Geometry: final body of the model. Coordinates: model frame, mm. Face numbers are marked on the shaded views. Give positions to 0.01 mm unless a question says otherwise; leave off trailing zeros. Loops run counter-clockwise (first coordinate to the right, second up) from the corner with the lowest first, then second, coordinate; pieces in that order, holes last.
1. Material intervals for line 1 along Y through (x, z) = (231, 31.5); line 2 along Z through (x, y) = (208, 17); line 3 along Y through (x, z) = (153.5, 22), sorted ascending.
2. Section C-C, the plane x = 138. Output: boundary loops of the cut face in (y, z), then the cut area to 3 significant figures.
3. First-contact query: P1, Ø8, axis at x = 198.77, y = 19.99, coming from the +Z side; P2, Ø7, axis at x = 132.5, z = 25, coming from the +Y side; P3, Ø22, axis at x = 86, y = 18.5, coming from the +Z side. Flat tips, straight axial feed; report the tip coordinate or a pass-through.
4. Draft query along Y for the marked faces 1, 2, 3 and 4. Return one class per face: +Y half, -Y half, draft (parallel to the pull), parting line (faces both ways), or undercut.
5. Section A-A, the plane x = 31.5. Output: boundary loops of the cut face in (y, z), then the cut area to 3 significant figures.
6. Section B-B, the plane z = 42. Output: boundary loops of the cut face in (x, y), then the cut area to 3 significant figures.
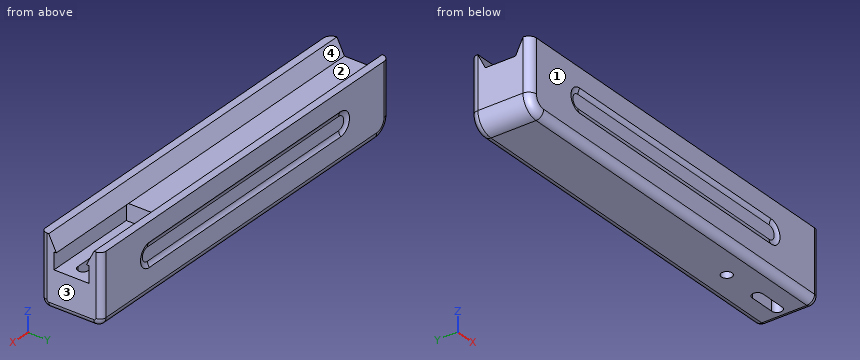
from build123d import *

# Parameters (mm, degrees)
SKETCH1_W           = 256.8448
SKETCH1_H           = 39.99738
BOSS_EXTRUDE1_DEPTH = 45.9994
CUT_EXTRUDE1_DEPTH  = 264.979140264
SKETCH3_W           = 11.01852
SKETCH3_H           = 22.9997
CUT_EXTRUDE2_DEPTH  = 67.27444
SKETCH4_R           = 3.49631
CUT_EXTRUDE3_DEPTH  = 262.138061298
CUT_EXTRUDE4_DEPTH  = 262.138061298
SKETCH6_W           = 45.9994
SKETCH6_H           = 39.99738
CUT_EXTRUDE5_DEPTH  = 3.81
FILLET1_R           = 3.81
FILLET2_R           = 11.43
FILLET3_R           = 5.08
CUT_EXTRUDE6_DEPTH  = 1.27
FILLET4_R           = 5.08
CUT_EXTRUDE7_DEPTH  = 1.27
FILLET5_R           = 5.08


with BuildPart() as part:
    # Sketch1 → Boss-Extrude1 (new body)
    with BuildSketch(Plane.XY):
        with Locations((128.4224, 19.99869)):
            Rectangle(SKETCH1_W, SKETCH1_H)
    extrude(amount=BOSS_EXTRUDE1_DEPTH)

    # Sketch2 → Cut-Extrude1 (cut, through all)
    with BuildSketch(Plane(origin=(256.8448, 0, 0), x_dir=(0, 0, -1), z_dir=(1, 0, 0))):
        Polygon((-35.99942, 9.99998), (-45.9994, 4.99872), (-45.9994, 34.99866), (-35.99942, 29.99994), align=None)
    extrude(amount=-CUT_EXTRUDE1_DEPTH, mode=Mode.SUBTRACT)

    # Sketch3 → Cut-Extrude2 (cut)
    with BuildSketch(Plane(origin=(256.8448, 0, 0), x_dir=(0, 0, -1), z_dir=(1, 0, 0))):
        with Locations((-30.49016, 19.99361)):
            Rectangle(SKETCH3_W, SKETCH3_H)
    extrude(amount=-CUT_EXTRUDE2_DEPTH, mode=Mode.SUBTRACT)

    # Sketch4 → Cut-Extrude3 (cut, through all)
    with BuildSketch(Plane.XY.offset(24.9809)):
        with Locations((198.77278, 19.99361)):
            Circle(SKETCH4_R)
    extrude(amount=-CUT_EXTRUDE3_DEPTH, mode=Mode.SUBTRACT)

    # Sketch5 → Cut-Extrude4 (cut, through all)
    with BuildSketch(Plane.XY.offset(24.9809)):
        with BuildLine():
            Line((242.77828, 23.48611), (225.78568, 23.48611))
            ThreePointArc((225.78568, 23.48611), (222.29318, 19.99361), (225.78568, 16.50111))
            Line((225.78568, 16.50111), (242.77828, 16.50111))
            ThreePointArc((242.77828, 16.50111), (246.27078, 19.99361), (242.77828, 23.48611))
        make_face()
    extrude(amount=-CUT_EXTRUDE4_DEPTH, mode=Mode.SUBTRACT)

    # Sketch6 → Cut-Extrude5 (cut)
    with BuildSketch(Plane(origin=(256.8448, 0, 0), x_dir=(0, 0, -1), z_dir=(1, 0, 0))):
        with Locations((-22.9997, 19.99869)):
            Rectangle(SKETCH6_W, SKETCH6_H)
    extrude(amount=-CUT_EXTRUDE5_DEPTH, mode=Mode.SUBTRACT)

    # Fillet1
    fillet1_edges = [part.edges().sort_by_distance(p)[0] for p in [
        (253.0348, 19.99869, 0),
        (253.0348, 0, 22.9997),
        (253.0348, 39.99738, 22.9997),
    ]]
    fillet(fillet1_edges, radius=FILLET1_R)

    # Fillet2
    fillet2_edges = [part.edges().sort_by_distance(p)[0] for p in [
        (0, 19.99869, 0),
    ]]
    fillet(fillet2_edges, radius=FILLET2_R)

    # Fillet3
    # the kernel refuses this fillet: 5.08 mm, written as the material it takes off along each edge
    with BuildSketch(Plane(origin=(253.0348, 34.91738, 5.08), x_dir=(0, 0, -1), z_dir=(0, -1, 0))) as fillet3_piece_1:
        with BuildLine():
            CenterArc((1.27, -3.81), 3.81, 0, 90)
            Line((5.08, -3.81), (5.08, 0))
            Line((5.08, 0), (1.27, 0))
        make_face()
    revolve(axis=Axis((253.0348, 34.91738, 5.08), (1, 0, 0)), revolution_arc=90, mode=Mode.SUBTRACT)
    with BuildSketch(Plane(origin=(253.0348, 5.08, 5.08), x_dir=(0, -1, 0), z_dir=(0, 0, 1))) as fillet3_piece_2:
        with BuildLine():
            CenterArc((1.27, -3.81), 3.81, 0, 90)
            Line((5.08, -3.81), (5.08, 0))
            Line((5.08, 0), (1.27, 0))
        make_face()
    revolve(axis=Axis((253.0348, 5.08, 5.08), (1, 0, 0)), revolution_arc=90, mode=Mode.SUBTRACT)
    with BuildSketch(Plane(origin=(0, 0, 11.43), x_dir=(1, 0, 0), z_dir=(0, 0, 1)), Plane(origin=(0, 39.99738, 11.43), x_dir=(0, -1, 0), z_dir=(0, 0, 1))) as fillet3_piece_3:
        with BuildLine():
            CenterArc((FILLET3_R, FILLET3_R), FILLET3_R, 180, 90)
            Line((0, FILLET3_R), (0, 0))
            Line((0, 0), (FILLET3_R, 0))
        make_face()
    extrude(amount=47.2694, mode=Mode.SUBTRACT)
    with BuildSketch(Plane(origin=(11.43, 0, 11.43), x_dir=(0, 0, -1), z_dir=(1, 0, 0))) as fillet3_piece_4:
        with BuildLine():
            CenterArc((11.43 - FILLET3_R, FILLET3_R), FILLET3_R, 270, 90)
            Line((11.43, FILLET3_R), (11.43, 0))
            Line((11.43, 0), (11.43 - FILLET3_R, 0))
        make_face()
    revolve(axis=Axis((11.43, 0, 11.43), (0, 1, 0)), revolution_arc=90, mode=Mode.SUBTRACT)
    with BuildSketch(Plane(origin=(11.43, 39.99738, 11.43), x_dir=(0, 0, -1), z_dir=(1, 0, 0))) as fillet3_piece_5:
        with BuildLine():
            CenterArc((11.43 - FILLET3_R, -FILLET3_R), FILLET3_R, 0, 90)
            Line((11.43 - FILLET3_R, 0), (11.43, 0))
            Line((11.43, 0), (11.43, -FILLET3_R))
        make_face()
    revolve(axis=Axis((11.43, 39.99738, 11.43), (0, 1, 0)), revolution_arc=90, mode=Mode.SUBTRACT)
    with BuildSketch(Plane(origin=(11.43, 0, 0), x_dir=(0, 0, 1), z_dir=(1, 0, 0))) as fillet3_piece_6:
        with BuildLine():
            CenterArc((FILLET3_R, -FILLET3_R), FILLET3_R, 90, 90)
            Line((0, -FILLET3_R), (0, 0))
            Line((0, 0), (FILLET3_R, 0))
        make_face()
    extrude(amount=241.6048, mode=Mode.SUBTRACT)
    with BuildSketch(Plane(origin=(253.0348, 39.99738, 0), x_dir=(0, -1, 0), z_dir=(-1, 0, 0))) as fillet3_piece_7:
        with BuildLine():
            CenterArc((FILLET3_R, FILLET3_R), FILLET3_R, 180, 90)
            Line((0, FILLET3_R), (0, 0))
            Line((0, 0), (FILLET3_R, 0))
        make_face()
    extrude(amount=241.6048, mode=Mode.SUBTRACT)

    # Sketch7 → Cut-Extrude6 (cut)
    with BuildSketch(Plane(origin=(0, 39.99738, 0), x_dir=(1, 0, 0), z_dir=(0, 1, 0))):
        with BuildLine():
            Line((211.1248, -33.2994), (43.18, -33.2994))
            ThreePointArc((43.18, -33.2994), (35.4203, -25.5397), (43.18, -17.78))
            Line((43.18, -17.78), (211.1248, -17.78))
            ThreePointArc((211.1248, -17.78), (218.8845, -25.5397), (211.1248, -33.2994))
        make_face()
    extrude(amount=-CUT_EXTRUDE6_DEPTH, mode=Mode.SUBTRACT)

    # Fillet4
    # the kernel refuses this fillet: 5.08 mm, written as the material it adds along each edge
    with BuildSketch(Plane(origin=(211.1248, 38.72738, 33.2994), x_dir=(0, 1, 0), z_dir=(-1, 0, 0)), Plane(origin=(43.18, 38.72738, 17.78), x_dir=(0, 1, 0), z_dir=(1, 0, 0))) as fillet4_piece_1:
        with BuildLine():
            CenterArc((5.08, 3.360104165), FILLET4_R, 180, 41.409622109)
            Line((0, 3.360104165), (-0.1016, 3.360104165))
            Line((-0.1016, 3.360104165), (-0.1016, 0))
            Line((-0.1016, 0), (0, -0.1016))
            ThreePointArc((0, -0.1016), (0.635, -0.1016), (1.1938, -0.067202083))
            Line((1.1938, -0.067202083), (1.27, 0))
        make_face()
    extrude(amount=167.9448)
    with BuildSketch(Plane(origin=(43.18, 38.72738, 25.5397), x_dir=(0, 0, 1), z_dir=(1, 0, 0))) as fillet4_piece_2:
        with BuildLine():
            CenterArc((4.399595835, -5.08), FILLET4_R, 48.590377891, 41.409622109)
            Line((4.399595835, 0), (4.399595835, 0.1016))
            Line((4.399595835, 0.1016), (7.7597, 0.1016))
            Line((7.7597, 0.1016), (7.8613, 0))
            ThreePointArc((7.8613, 0), (7.8613, -0.635), (7.826902083, -1.1938))
            Line((7.826902083, -1.1938), (7.7597, -1.27))
        make_face()
    revolve(axis=Axis((43.18, 38.72738, 25.5397), (0, -1, 0)), revolution_arc=180)
    with BuildSketch(Plane(origin=(211.1248, 38.72738, 25.5397), x_dir=(0, 0, -1), z_dir=(-1, 0, 0))) as fillet4_piece_3:
        with BuildLine():
            CenterArc((4.399595835, -5.08), FILLET4_R, 48.590377891, 41.409622109)
            Line((4.399595835, 0), (4.399595835, 0.1016))
            Line((4.399595835, 0.1016), (7.7597, 0.1016))
            Line((7.7597, 0.1016), (7.8613, 0))
            ThreePointArc((7.8613, 0), (7.8613, -0.635), (7.826902083, -1.1938))
            Line((7.826902083, -1.1938), (7.7597, -1.27))
        make_face()
    revolve(axis=Axis((211.1248, 38.72738, 25.5397), (0, -1, 0)), revolution_arc=180)

    # Sketch8 → Cut-Extrude7 (cut)
    with BuildSketch(Plane.XZ):
        with BuildLine():
            Line((43.18, 33.2994), (211.1248, 33.2994))
            ThreePointArc((211.1248, 33.2994), (218.8845, 25.5397), (211.1248, 17.78))
            Line((211.1248, 17.78), (43.18, 17.78))
            ThreePointArc((43.18, 17.78), (35.4203, 25.5397), (43.18, 33.2994))
        make_face()
    extrude(amount=-CUT_EXTRUDE7_DEPTH, mode=Mode.SUBTRACT)

    # Fillet5
    # the kernel refuses this fillet: 5.08 mm, written as the material it adds along each edge
    with BuildSketch(Plane(origin=(43.18, 1.27, 33.2994), x_dir=(0, -1, 0), z_dir=(1, 0, 0)), Plane(origin=(211.1248, 1.27, 17.78), x_dir=(0, -1, 0), z_dir=(-1, 0, 0))) as fillet5_piece_1:
        with BuildLine():
            CenterArc((5.08, 3.360104165), FILLET5_R, 180, 41.409622109)
            Line((0, 3.360104165), (-0.1016, 3.360104165))
            Line((-0.1016, 3.360104165), (-0.1016, 0))
            Line((-0.1016, 0), (0, -0.1016))
            ThreePointArc((0, -0.1016), (0.635, -0.1016), (1.1938, -0.067202083))
            Line((1.1938, -0.067202083), (1.27, 0))
        make_face()
    extrude(amount=167.9448)
    with BuildSketch(Plane(origin=(211.1248, 1.27, 25.5397), x_dir=(0, 0, 1), z_dir=(-1, 0, 0))) as fillet5_piece_2:
        with BuildLine():
            CenterArc((4.399595835, -5.08), FILLET5_R, 48.590377891, 41.409622109)
            Line((4.399595835, 0), (4.399595835, 0.1016))
            Line((4.399595835, 0.1016), (7.7597, 0.1016))
            Line((7.7597, 0.1016), (7.8613, 0))
            ThreePointArc((7.8613, 0), (7.8613, -0.635), (7.826902083, -1.1938))
            Line((7.826902083, -1.1938), (7.7597, -1.27))
        make_face()
    revolve(axis=Axis((211.1248, 1.27, 25.5397), (0, 1, 0)), revolution_arc=180)
    with BuildSketch(Plane(origin=(43.18, 1.27, 25.5397), x_dir=(0, 0, -1), z_dir=(1, 0, 0))) as fillet5_piece_3:
        with BuildLine():
            CenterArc((4.399595835, -5.08), FILLET5_R, 48.590377891, 41.409622109)
            Line((4.399595835, 0), (4.399595835, 0.1016))
            Line((4.399595835, 0.1016), (7.7597, 0.1016))
            Line((7.7597, 0.1016), (7.8613, 0))
            ThreePointArc((7.8613, 0), (7.8613, -0.635), (7.826902083, -1.1938))
            Line((7.826902083, -1.1938), (7.7597, -1.27))
        make_face()
    revolve(axis=Axis((43.18, 1.27, 25.5397), (0, 1, 0)), revolution_arc=180)


solid = part.part
Answers below:
1. line 1: y = 0 to 8.49, 31.49 to 40
1. line 2: z = 0 to 24.98
1. line 3: y = 1.27 to 38.73
2. outline: (0, 5.08) arc R5.08 ccw to (5.08, 0) - (34.92, 0) arc R5.08 ccw to (40, 5.08) - (40, 17.78) arc R5.08 cw to (38.73, 21.14) - (38.73, 29.94) arc R5.08 cw to (40, 33.3) - (40, 46) - (35, 46) - (30, 36) - (10, 36) - (5, 46) - (0, 46) - (0, 33.3) arc R5.08 cw to (1.27, 29.94) - (1.27, 21.14) arc R5.08 cw to (0, 17.78) - close
2. area: 1,540 mm2
3. P1: stops at z = 24.98
3. P2: stops at y = 38.73
3. P3: stops at z = 41
4. face 1: -Y half
4. face 2: undercut
4. face 3: draft
4. face 4: undercut
5. outline: (0, 5.08) arc R5.08 ccw to (5.08, 0) - (34.92, 0) arc R5.08 ccw to (40, 5.08) - (40, 46) - (35, 46) - (30, 36) - (10, 36) - (5, 46) - (0, 46) - close
5. area: 1,580 mm2
6. outline: (0, 5.08) arc R5.08 ccw to (5.08, 0) - (249.22, 0) arc R3.81 ccw to (253.03, 3.81) - (253.03, 7) - (0, 7) - close; (0, 33) - (253.03, 33) - (253.03, 36.19) arc R3.81 ccw to (249.22, 40) - (5.08, 40) arc R5.08 ccw to (0, 34.92) - close
6. area: 3,520 mm2
